Can you work these out from the model? Positions are in its coordinate system, mm. Face numbers are marked on the shaded views. Coordinates: 2 decimals unless noted, no trailing zeros. Order: outer loops, then holes, each group sorted by start corner. A loop starts at its lowest first (then second) coordinate and runs counter-clockwise, first axis right, second up. Notation, with made-up numbers: (28.25, 7) -> (77.25, 7) arc R25 ccw to (77.25, 42) -> close; hole circle Ø4 at (15, 57.25). An arc over 180 degrees is marked (long way). Write item = value, one per line. Start each with the question number.
from build123d import *

# Parameters (mm, degrees)
SKETCH_1_R      = 2.44
EXTRUDE_1_DEPTH = 4
FILLET_2_R      = 1
FILLET_4_R      = 1
FILLET_5_R      = 1
FILLET_6_R      = 1


with BuildPart() as part:
    # 草图1 → 凸台-拉伸1 (new body)
    with BuildSketch(Plane.XY):
        with BuildLine():
            Line((-29.190524981, -5.5), (29.190524981, -5.5))
            ThreePointArc((29.190524981, -5.5), (43, 0), (29.190524981, 5.5))
            Line((29.190524981, 5.5), (-29.190524981, 5.5))
            ThreePointArc((-29.190524981, 5.5), (-43, 0), (-29.190524981, -5.5))
        make_face()
        with Locations((35, 0)):
            Circle(SKETCH_1_R, mode=Mode.SUBTRACT)
        with Locations((-35, 0)):
            Circle(SKETCH_1_R, mode=Mode.SUBTRACT)
        with BuildLine():
            ThreePointArc((22.5, -2.540734009), (25.040734009, 0), (22.5, 2.540734009))
            Line((22.5, 2.540734009), (-22.5, 2.540734009))
            ThreePointArc((-22.5, 2.540734009), (-25.040734009, 0), (-22.5, -2.540734009))
            Line((-22.5, -2.540734009), (22.5, -2.540734009))
        make_face(mode=Mode.SUBTRACT)
    extrude(amount=EXTRUDE_1_DEPTH)

    # 圆角2
    fillet_2_edges = [part.edges().sort_by_distance(p)[0] for p in [
        (-29.190524981, 5.5, 2),
    ]]
    fillet(fillet_2_edges, radius=FILLET_2_R)

    # 圆角4
    fillet_4_edges = [part.edges().sort_by_distance(p)[0] for p in [
        (-29.190524981, -5.5, 2),
    ]]
    fillet(fillet_4_edges, radius=FILLET_4_R)

    # 圆角5
    fillet_5_edges = [part.edges().sort_by_distance(p)[0] for p in [
        (29.190524981, 5.5, 2),
    ]]
    fillet(fillet_5_edges, radius=FILLET_5_R)

    # 圆角6
    fillet_6_edges = [part.edges().sort_by_distance(p)[0] for p in [
        (29.190524981, -5.5, 2),
    ]]
    fillet(fillet_6_edges, radius=FILLET_6_R)


solid = part.part
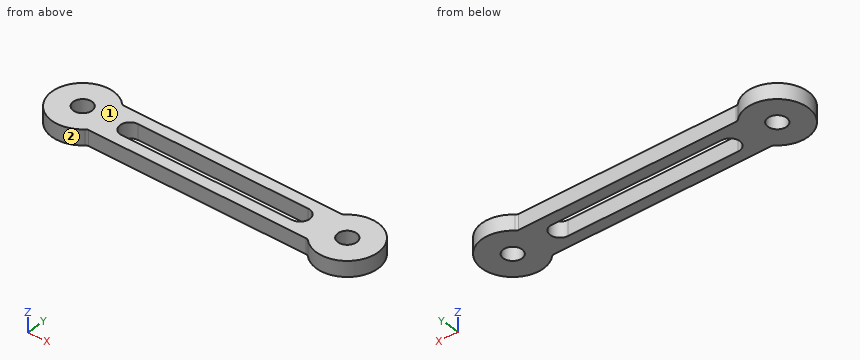
(1) Imagine slicing it at B-B (y = 0). Write out the boundary of the cut face in (x, z).
(2) For P1, Ø2, axis at x = 16.5, z = 1, coming from the +Y side; P2, Ø4.5, axis at x = -35, y = 0, coming from the -Z side; P3, Ø2, axis at x = 21.5, z = 1, coming from the -Y side; P4, Ø2, axis at y = -4.5, z = 0.5, coming from the -X side, each with a flat end and sliding along its axis, tell me the tip position at first contact or that it passes through.
(3) Thinking about a two-plate mould opening in X: for the marked faces 1 and 2, which applies, +X half, -X half, draft (parallel to the pull), parting line (faces both ways), or undercut?
(4) Imagine slicing it at C-C (z = 2.55). Write out the boundary of the cut face in (x, y).
(5) Imagine slicing it at D-D (x = 20.5). Write out the boundary of the cut face in (y, z), plus the area to 3 significant figures.
(6) Imagine slicing it at A-A (x = -35). Write out the boundary of the cut face in (y, z).
(7) If I drill on L1, parallel to X at y = 0.25, z = 1.65; L2, parallel to X at y = -2, z = 2.3; L3, parallel to Y at x = 22, z = 0.7, over which ranges is the centre line in solid material (lowest first)? Write a range as from..to.
Result set:
q1.outline = (-43, 0) -> (-37.44, 0) -> (-37.44, 4) -> (-43, 4) -> close; (-32.56, 0) -> (-25.04, 0) -> (-25.04, 4) -> (-32.56, 4) -> close; (25.04, 0) -> (32.56, 0) -> (32.56, 4) -> (25.04, 4) -> close; (37.44, 0) -> (43, 0) -> (43, 4) -> (37.44, 4) -> close
q2.P1 = 5.5
q2.P2 = through
q2.P3 = -5.5
q2.P4 = -42.19
q3.face_1 = draft
q3.face_2 = undercut
q4.outline = (-29.47, -5.78) arc R1 cw to (-28.78, -5.5) -> (28.78, -5.5) arc R1 cw to (29.47, -5.78) arc R8 ccw (long way) to (29.47, 5.78) arc R1 cw to (28.78, 5.5) -> (-28.78, 5.5) arc R1 cw to (-29.47, 5.78) arc R8 ccw (long way) to start; hole circle Ø4.88 at (-35, 0); hole (-22.5, -2.54) -> (22.5, -2.54) arc R2.54 ccw to (22.5, 2.54) -> (-22.5, 2.54) arc R2.54 ccw to start; hole circle Ø4.88 at (35, 0)
q5.outline = (-5.5, 0) -> (-2.54, 0) -> (-2.54, 4) -> (-5.5, 4) -> close; (2.54, 0) -> (5.5, 0) -> (5.5, 4) -> (2.54, 4) -> close
q5.area = 23.7 mm2
q6.outline = (-8, 0) -> (-2.44, 0) -> (-2.44, 4) -> (-8, 4) -> close; (2.44, 0) -> (8, 0) -> (8, 4) -> (2.44, 4) -> close
q7.L1 = -43..-37.43, -32.57..-25.03, 25.03..32.57, 37.43..43
q7.L2 = -42.75..-36.4, -33.6..-24.07, 24.07..33.6, 36.4..42.75
q7.L3 = -5.5..-2.54, 2.54..5.5
